Verification items for the finished model (mm, model axes). A direction names the side the tool comes from. Round coordinates to 2 decimals unless told otherwise and drop trailing zeros. Write each loop counter-clockwise with the first axis right and the second up, starting at its lowest first coordinate (ties: lowest second). Pieces come first, ordered by that corner, then holes. Notation, with made-up numbers: (76.5, 72) -> (87.5, 72) arc R30 cw to (87.5, 94) -> close; hole circle Ø10 at (61.25, -21). An arc over 180 degrees is marked (long way). Answer as a JSON object with one key per item and string values. Group by question number.
(1) Draft check along Z on faces 5 (the face through (-3.76, -5.77, 26.92)), 6 (the face through (0, 3, 22)), 7 (the face through (-7, -6, 25.8)). Enter one of: released by +Z, released by -Z, zero draft, split by the parting line, or undercut.
(2) Sectioned sample at B-B on z = 15. Record the cut outline in (x, y).
(3) Gauge pin test, flat ends, axial feed: pin 1 Ø2.5 at (y, z) = (2, 8.5) entering from +X; pin 2 Ø2.5 at (x, y) = (3.5, -6) entering from -Z; pin 3 Ø6 at (x, z) = (-3, -1.5) entering from -Y. Record the tip position at first contact, or that the pin passes through.
(4) Sectioned sample at A-A on x = 0. Count the separate pieces of the cut face and the enclosed holes in it, and give its area (3 significant figures).
(5) Sectioned sample at C-C on y = -3.25. Record the cut outline in (x, z).
(6) Sectioned sample at D-D on y = -6. Record the cut outline in (x, z).
(7) Set-up check for faces 1 (the face through (-3, 2, 26)), 2 (the face through (-6.95, 1.48, 3.89)), 3 (the face through (6.953, 1.479, 3.88)), 4 (the face through (-6.91, 3.51, 18.64)): record each of +Z, -Z, +X, -X, +Y, -Y from which the full face is reachable in a straight line by a thin tool's end or side.
(8) Scan lines: L1, parallel to X at y = 0.4, z = 0; L2, parallel to X at y = -0.5, z = 0; L3, parallel to Y at x = -4, z = 19. Record each from-to range of solid material in increasing order. Write a range as from..to.
```python
from build123d import *
from build123d.topology import SkipClean

# Parameters (mm, degrees)
EXTRUDE_1_DEPTH     = 4
EXTRUDE_3_DEPTH     = 6
CHAMFER_1_SIZE      = 3
CUT_EXTRUDE_2_DEPTH = 2.5
CUT_EXTRUDE_3_REACH = 32.453
SKETCH_7_R          = 1.35
SKETCH_8_R          = 6
EXTRUDE_4_DEPTH     = 1
FILLET_1_R          = 0.5
SKETCH_9_R          = 5
CUT_EXTRUDE_4_DEPTH = 3
SKETCH_10_R         = 3.55
CUT_EXTRUDE_5_DEPTH = 3.6
CUT_EXTRUDE_6_DEPTH = 0.8
CUT_EXTRUDE_7_DEPTH = 32.283541999
FILLET_2_R          = 2
CHAMFER_2_SIZE      = 1


with BuildPart() as part:
    # ｽｹｯﾁ1 → ﾎﾞｽ - 押し出し1 (new body)
    with BuildSketch(Plane(origin=(0, 0, 0), x_dir=(1, 0, 0), z_dir=(0, 1, 0))):
        with BuildLine():
            Line((-7.9, 0), (-7.9, -28))
            Line((-7.9, -28), (7.9, -28))
            Line((7.9, -28), (7.9, 0))
            ThreePointArc((7.9, 0), (0, 7.9), (-7.9, 0))
        make_face()
    extrude(amount=EXTRUDE_1_DEPTH)

    # ｽｹｯﾁ4 → ﾎﾞｽ - 押し出し3 (add)
    with BuildSketch(Plane.XY.offset(28)):
        Polygon((-7, -7.5), (-4.5, -7.5), (-3, -4), (3, -4), (4.5, -7.5), (7, -7.5), (7.9, -4), (7.9, 0), (-7.9, 0), (-7.9, -4), align=None)
    extrude(amount=-EXTRUDE_3_DEPTH)

    # 面取り1
    chamfer_1_edges = [part.edges().sort_by_distance(p)[0] for p in [
        (0, 4, 28),
    ]]
    chamfer(chamfer_1_edges, length=CHAMFER_1_SIZE)

    # ｽｹｯﾁ6 → ｶｯﾄ - 押し出し2 (cut)
    with BuildSketch(Plane(origin=(0, 4, 0), x_dir=(1, 0, 0), z_dir=(0, 1, 0))):
        with BuildLine():
            Line((-3, -25), (-3, -29))
            Line((-3, -29), (3, -29))
            Line((3, -29), (3, -25))
            ThreePointArc((3, -25), (0, -22), (-3, -25))
        make_face()
    extrude(amount=-CUT_EXTRUDE_2_DEPTH, mode=Mode.SUBTRACT)

    # ｽｹｯﾁ7 → ｶｯﾄ - 押し出し3 (cut, up to next)
    with BuildSketch(Plane(origin=(0, 1.5, 0), x_dir=(1, 0, 0), z_dir=(0, 1, 0)), mode=Mode.PRIVATE) as cut_extrude_3_sk1:
        with Locations(Location((0, -25, 0), (0, 0, 270))):
            Circle(SKETCH_7_R)
    cut_extrude_3_tool1 = extrude(cut_extrude_3_sk1.sketch, amount=-CUT_EXTRUDE_3_REACH, mode=Mode.PRIVATE) & part.part
    add(cut_extrude_3_tool1.solids().sort_by_distance((0, 1.5, 25))[0], mode=Mode.SUBTRACT)

    # ｽｹｯﾁ8 → ﾎﾞｽ - 押し出し4 (add)
    with BuildSketch(Plane.XZ):
        with Locations(Location((0, 0, 0), (0, 0, 90))):
            Circle(SKETCH_8_R)
    extrude(amount=EXTRUDE_4_DEPTH)

    # ﾌｨﾚｯﾄ1
    fillet_1_edges = [part.edges().sort_by_distance(p)[0] for p in [
        (0, 0, -6),
    ]]
    fillet(fillet_1_edges, radius=FILLET_1_R)

    # ｽｹｯﾁ9 → ｶｯﾄ - 押し出し4 (cut)
    with BuildSketch(Plane(origin=(0, 4, 0), x_dir=(1, 0, 0), z_dir=(0, 1, 0))):
        with Locations(Location((0, 0, 0), (0, 0, 270))):
            Circle(SKETCH_9_R)
    extrude(amount=-CUT_EXTRUDE_4_DEPTH, mode=Mode.SUBTRACT)

    # ｽｹｯﾁ10 → ｶｯﾄ - 押し出し5 (cut)
    with BuildSketch(Plane(origin=(0, 1, 0), x_dir=(1, 0, 0), z_dir=(0, 1, 0))):
        with Locations(Location((0, 0, 0), (0, 0, 270))):
            Circle(SKETCH_10_R)
    extrude(amount=-CUT_EXTRUDE_5_DEPTH, mode=Mode.SUBTRACT)

    # ｽｹｯﾁ11 → ｶｯﾄ - 押し出し6 (cut, symmetric)
    with BuildSketch(Plane.XY.offset(25)):
        Polygon((3, -4), (4.5, -7.5), (5.1, -7.5), (3.6, -4), align=None)
        Polygon((6.4, -7.5), (7, -7.5), (7.9, -4), (7.3, -4), align=None)
    cut_extrude_6 = extrude(amount=CUT_EXTRUDE_6_DEPTH, both=True, mode=Mode.SUBTRACT)

    # ﾐﾗｰ1: ｶｯﾄ - 押し出し6 across plane
    add(cut_extrude_6.mirror(Plane(origin=(0, 0, 0), x_dir=(0, 0, 1), z_dir=(1, 0, 0))), mode=Mode.SUBTRACT)

    # ｽｹｯﾁ12 → ｶｯﾄ - 押し出し7 (cut, through all)
    with SkipClean():  # the faces are left unmerged after this step: merging them gives an invalid solid
        with BuildSketch(Plane(origin=(0, 4, 0), x_dir=(1, 0, 0), z_dir=(0, 1, 0))):
            with BuildLine():
                Line((-7.9, 0), (-7.9, -20))
                Line((-7.9, -20), (-6.9, -17))
                Line((-6.9, -17), (-6.9, -3.847076812))
                ThreePointArc((-6.9, -3.847076812), (-7.645913941, -1.987460691), (-7.9, 0))
            make_face()
        cut_extrude_7 = extrude(amount=-CUT_EXTRUDE_7_DEPTH, mode=Mode.SUBTRACT)

    # ﾐﾗｰ2: ｶｯﾄ - 押し出し7 across plane
    with SkipClean():  # the faces are left unmerged after this step: merging them gives an invalid solid
        add(cut_extrude_7.mirror(Plane(origin=(0, 0, 0), x_dir=(0, 0, 1), z_dir=(1, 0, 0))), mode=Mode.SUBTRACT)

    # ﾌｨﾚｯﾄ2
    fillet_2_edges = [part.edges().sort_by_distance(p)[0] for p in [
        (-6.9, 2, 3.847076812),
        (-6.9, 2, 17),
        (-7.9, 2, 20),
        (6.9, 2, 3.847076812),
        (7.9, 2, 20),
        (6.9, 2, 17),
    ]]
    fillet(fillet_2_edges, radius=FILLET_2_R)

    # 面取り2
    chamfer_2_edges = [part.edges().sort_by_distance(p)[0] for p in [
        (-7.9, 4, 22.66227766),
        (0, 4, -7.9),
        (7.9, 4, 22.66227766),
        (0, 0, 22),
        (-7.874174915, 4, 20.004190834),
        (-7.4, 4, 18.5),
        (-6.925825085, 4, 16.995809166),
        (-6.9, 4, 10.505670679),
        (-6.951159371, 4, 3.886430103),
        (6.951159371, 4, 3.886430103),
        (6.9, 4, 10.505670679),
        (6.925825085, 4, 16.995809166),
        (7.4, 4, 18.5),
        (7.874174915, 4, 20.004190834),
    ]]
    chamfer(chamfer_2_edges, length=CHAMFER_2_SIZE)


solid = part.part
```
Computed values:
{
 "1": {"face 5": "zero draft", "face 6": "released by +Z", "face 7": "undercut"},
 "2": {"outline": "(-6.9, 0) -> (6.9, 0) -> (6.9, 3) -> (5.9, 4) -> (-5.9, 4) -> (-6.9, 3) -> close"},
 "3": {"pin 1": "x = 6.9", "pin 2": "z = 22", "pin 3": "y = -1"},
 "4": {"separate pieces": "3", "enclosed holes": "0", "area": "106 mm2"},
 "5": {"outline": "(-7.9, 22) -> (7.9, 22) -> (7.9, 28) -> (-7.9, 28) -> close; hole circle Ø2.7 at (0, 25)"},
 "6": {"outline": "(-7.39, 22) -> (-3.86, 22) -> (-3.86, 24.2) -> (-4.46, 24.2) -> (-4.46, 25.8) -> (-3.86, 25.8) -> (-3.86, 28) -> (-7.39, 28) -> (-7.39, 25.8) -> (-6.79, 25.8) -> (-6.79, 24.2) -> (-7.39, 24.2) -> close; (3.86, 22) -> (7.39, 22) -> (7.39, 24.2) -> (6.79, 24.2) -> (6.79, 25.8) -> (7.39, 25.8) -> (7.39, 28) -> (3.86, 28) -> (3.86, 25.8) -> (4.46, 25.8) -> (4.46, 24.2) -> (3.86, 24.2) -> close"},
 "7": {"face 1": "+Z, +Y", "face 2": "-X, +Y, -Y", "face 3": "+X, +Y, -Y", "face 4": "-X, +Y"},
 "8": {"L1": "-7.9..-3.55, 3.55..7.9", "L2": "-6..-3.55, 3.55..6", "L3": "0..4"}
}
